Autodesk Inventor part; units mm, degrees
ref_plane "YZ Plane" through (0, 0, 0) normal (1, 0, 0) x (0, 1, 0)
ref_plane "XZ Plane" through (0, 0, 0) normal (0, 1, 0) x (-1, 0, 0)
ref_plane "XY Plane" through (0, 0, 0) normal (0, 0, 1) x (1, 0, 0)
sketch "Эскиз1" plane through (0, 0, 0) normal (0, 1, 0) x (-1, 0, 0)
  circle A0 centre (0, 0) radius 7.5
  dimension "d0" = 15
extrude "Выдавливание1" add sketch "Эскиз1" along normal blind 4
sketch "Эскиз2" plane through (0, 4, 0) normal (0, 1, 0) x (1, 0, 0)
  circle A0 centre (0, 0) radius 4
  dimension "d3" = 8
extrude "Выдавливание2" add sketch "Эскиз2" along normal blind 25
chamfer "Фаска1" distance 3.5 angle 45 1 edges at (7.5, 4, 0)
thread "Резьба1"
chamfer "Фаска2" distance 0.5 angle 45 1 edges at (-4, 29, 0)
sketch "Эскиз3" plane through (0, 0, 0) normal (0, -1, 0) x (1, 0, 0)
  line L0 (-5, -1) -> (5, -1)
  line L1 (5, -1) -> (5, 1)
  line L2 (5, 1) -> (-5, 1)
  line L3 (-5, 1) -> (-5, -1)
  line L4 (-5, -1) -> (5, 1) construction
  line L5 (5, -1) -> (-5, 1) construction
  line L6 (-1, -5) -> (1, -5)
  line L7 (1, -5) -> (1, 5)
  line L8 (1, 5) -> (-1, 5)
  line L9 (-1, 5) -> (-1, -5)
  line L10 (-1, -5) -> (1, 5) construction
  line L11 (1, -5) -> (-1, 5) construction
  point P0 (0, 0)
  dimension "d14" = 10
  dimension "d15" = 2
  dimension "d16" = 10
  dimension "d17" = 2
extrude "Выдавливание3" cut sketch "Эскиз3" against normal blind 2.5
properties part number "Винт М8х25 с потайной головкой" material "Сталь"
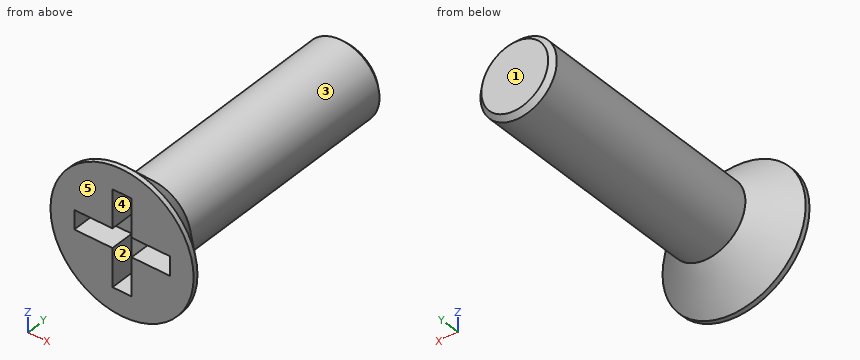
Work out the finished part from the listing and answer in its coordinate system (mm). Face numbers are marked on the shaded views. A direction names the side the tool comes from. Coordinates: 2 decimals unless noted, no trailing zeros. Loops run counter-clockwise (first coordinate to the right, second up) from the corner with the lowest first, then second, coordinate; pieces in that order, holes last. Notation, with made-up numbers: M 81,19 L 106,19 A28 ccw 106,50 Z; hole C 41,-2.75 d4. An arc over 180 degrees is marked long. Answer in a Markdown table with one row per item. Add a question column.
1. Find section C-C, the plane y = 24.5. Write down the section's boundary in (x, z), then the cut area to 3 significant figures.
2. The mould has two halves that part along Z. Classify the marked faces 3, 4 and 5: pulls with the +Z half, pulls with the -Z half, needs draft (parallel to the pull), parting line crosses it, or undercut.
3. A tool of negligible diameter and unlimited length cuts with its end or side. For the marked faces 1 and 2, from which of +Z, -Z, +X, -X, +Y, -Y can it reach the whole face along a straight path? Write none if from no direction.
4. Consider L1, parallel to Z at x = 0, y = 19.25; L2, parallel to Y at x = -1.5, z = 0.75; L3, parallel to X at y = 25.75, z = 2.25. Determine where each line is inside the solid, lowest interval first.
5. Flat-ended cylindrical pins translate along their axes: P1, Ø3, axis at x = 6, y = 4.5, coming from the -Z side; P2, Ø3, axis at x = 2.5, y = 10.5, coming from the -Z side; P3, Ø5, axis at x = 5, y = 18.5, coming from the +Z side; P4, Ø2, axis at x = 3.5, y = 0.5, coming from the -Z side. Find the tip coordinate at first contact, or state that the pin passes through.
Reported:
| question | item | result |
|---|---|---|
| 1 | outline | C 0,0 d8 |
| 1 | area | 50.3 mm^2 |
| 2 | face 3 | parting line crosses it |
| 2 | face 4 | undercut |
| 2 | face 5 | needs draft |
| 3 | face 1 | +Z, -Z, +X, -X, +Y |
| 3 | face 2 | -Y |
| 4 | L1 | z = -4 to 4 |
| 4 | L2 | y = 2.5 to 29 |
| 4 | L3 | x = -3.31 to 3.31 |
| 5 | P1 | passes through |
| 5 | P2 | stops at z = -3.87 |
| 5 | P3 | stops at z = 3.12 |
| 5 | P4 | stops at z = -7.07 |
